Check sheet for the drawn part. Datum: minimum x, y, z corner. Units: mm. Round coordinates to 2 decimals unless told otherwise and drop trailing zeros. Order: outer loops, then holes, each group sorted by start corner. A loop starts at its lowest first (then second) coordinate and runs counter-clockwise, first axis right, second up.
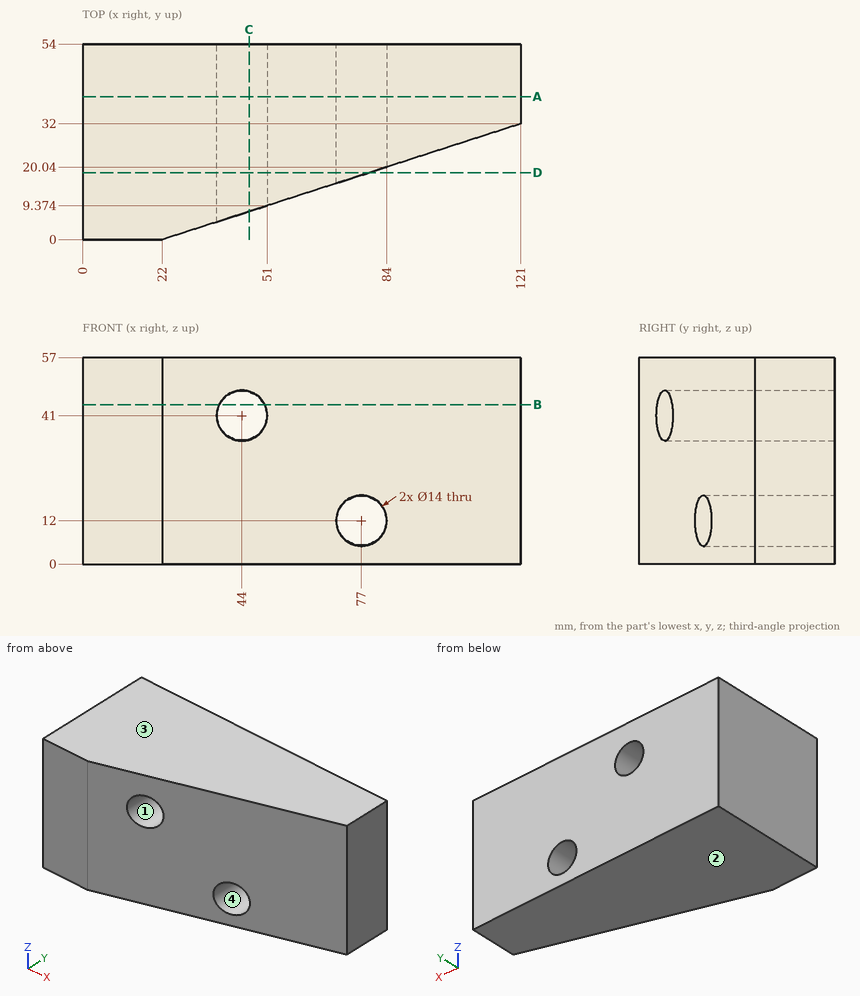
1) Draft check along Z on the marked faces 1, 2, 3 and 4. Enter one of: pulls with the +Z half, pulls with the -Z half, needs draft (parallel to the pull), parting line crosses it, or undercut.
2) Scan lines: line 1 (Z direction, x = 77, y = 39); line 2 (Z direction, x = 44, y = 17.5); line 3 (Y direction, x = 70, z = 13) (1 decimal). Record each from-to range of solid material in increasing order.
3) Sectioned sample at C-C on x = 46. Record the cut outline in (y, z), and give its area (3 significant figures).
4) Gauge pin test, flat ends, axial feed: pin 1 (5 mm diameter, centred on y = 24, z = 47.5, fed in from -X); pin 2 (11 mm diameter, centred on x = 44, z = 41, fed in from +Y); pin 3 (12 mm diameter, centred on x = 60, z = 43.5, fed in from -Y). Record the tip position at first contact, or that the pin passes through.
5) Sectioned sample at D-D on y = 18.5. Record the cut outline in (x, z) (1 decimal).
6) Sectioned sample at A-A on y = 39.5. Record the cut outline in (x, z), and give its area (3 significant figures).
7) Sectioned sample at B-B on z = 44. Record the cut outline in (x, y) (1 decimal), and give its area (3 significant figures).
Values found:
1. face 1: undercut
1. face 2: pulls with the -Z half
1. face 3: pulls with the +Z half
1. face 4: undercut
2. line 1: z = 0 to 5, 19 to 57
2. line 2: z = 0 to 34, 48 to 57
2. line 3: y = 15.5 to 54
3. outline: (7.76, 0) - (54, 0) - (54, 34.29) - (7.76, 34.29) - close; (7.76, 47.71) - (54, 47.71) - (54, 57) - (7.76, 57) - close
3. area: 2,020 mm2
4. pin 1: stops at x = 0
4. pin 2: passes through
4. pin 3: stops at y = 10.34
5. outline: (0, 0) - (79.2, 0) - (79.2, 5.4) arc R7 cw (long way) to (79.2, 18.6) - (79.2, 57) - (0, 57) - close; hole circle Ø14 at (44, 41)
6. outline: (0, 0) - (121, 0) - (121, 57) - (0, 57) - close; hole circle Ø14 at (44, 41); hole circle Ø14 at (77, 12)
6. area: 6,590 mm2
7. outline: (0, 0) - (22, 0) - (37.7, 5.1) - (37.7, 54) - (0, 54) - close; (50.3, 9.2) - (121, 32) - (121, 54) - (50.3, 54) - close
7. area: 4,360 mm2
